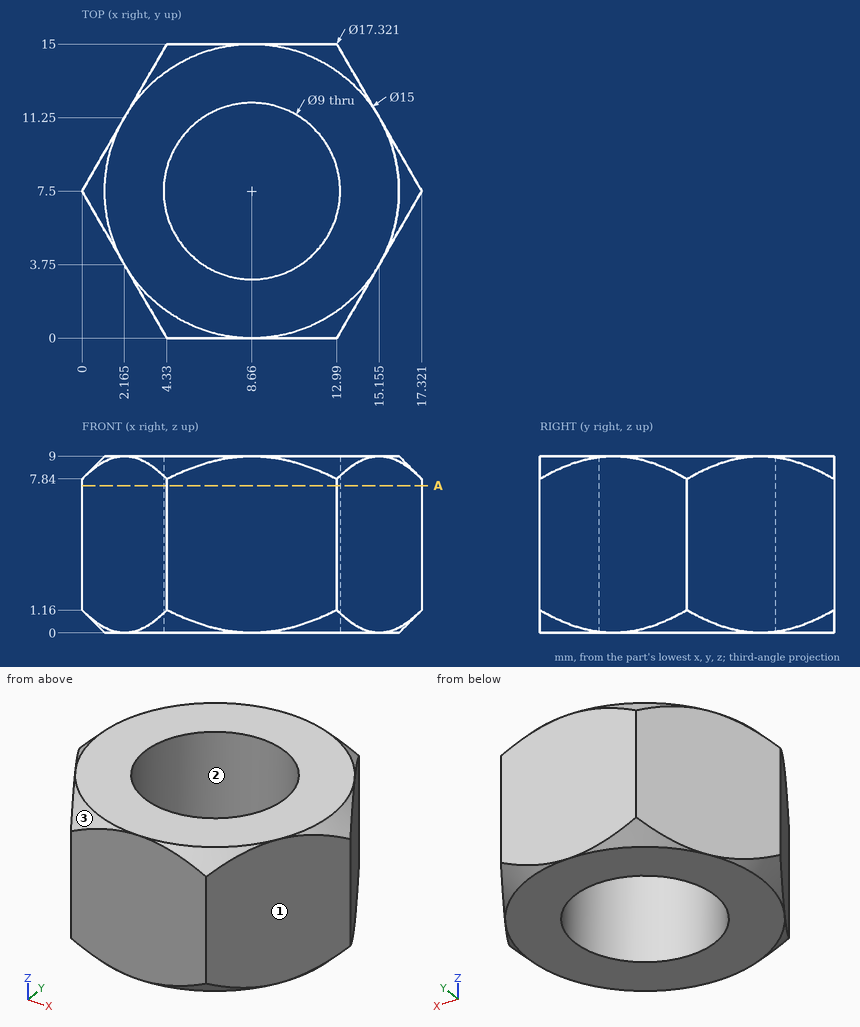
The drawing under review shows one solid part. Ordinate dimensions are in mm from its lowest x, y, z. Round coordinates to 2 decimals unless told otherwise and drop trailing zeros. Write each loop counter-clockwise with the first axis right and the second up, starting at its lowest first coordinate (ties: lowest second). Pieces come first, ordered by that corner, then holes. Notation, with made-up numbers: (52, 21.5) - (107, 21.5) arc R29 cw to (107, 49.5) - close; hole circle Ø7 at (65.5, 34). An arc over 180 degrees is marked (long way). One line per question, with ' | ' between items.
Item 1: For P1, Ø5, axis at y = 2.5, z = 7, coming from the +X side, flat-tipped, find the tip position at first contact; note if it passes through.
Resolved:
P1: stops at x = 15.88
Item 2: The part is to be moulded in two halves that separate along X. For the marked faces 1, 2 and 3, say which applies: pulls with the +X half, pulls with the -X half, needs draft (parallel to the pull), parting line crosses it, or undercut.
Resolved:
face 1: pulls with the +X half | face 2: undercut | face 3: pulls with the -X half
Item 3: To check wall thickness, follow probe 1 along Y at (x, z) = (8.5, 8.5); probe 2 along X at (y, z) = (6.75, 0.75) (1 decimal); probe 3 along Y at (x, z) = (10, 4.5) (1 decimal). State the ranges of each line that lie inside material, in increasing order.
Resolved:
probe 1: y = 0 to 3, 12 to 15 | probe 2: x = 0.4 to 4.2, 13.1 to 16.9 | probe 3: y = 0 to 3.2, 11.8 to 15
Item 4: Add section A-A, the plane z = 7.5. Give the boundary of the cut face in (x, y), then the cut area to 3 significant figures.
Resolved:
outline: (0, 7.5) - (4.33, 0) - (12.99, 0) - (17.32, 7.5) - (12.99, 15) - (4.33, 15) - close; hole circle Ø9 at (8.66, 7.5) | area: 131 mm2
